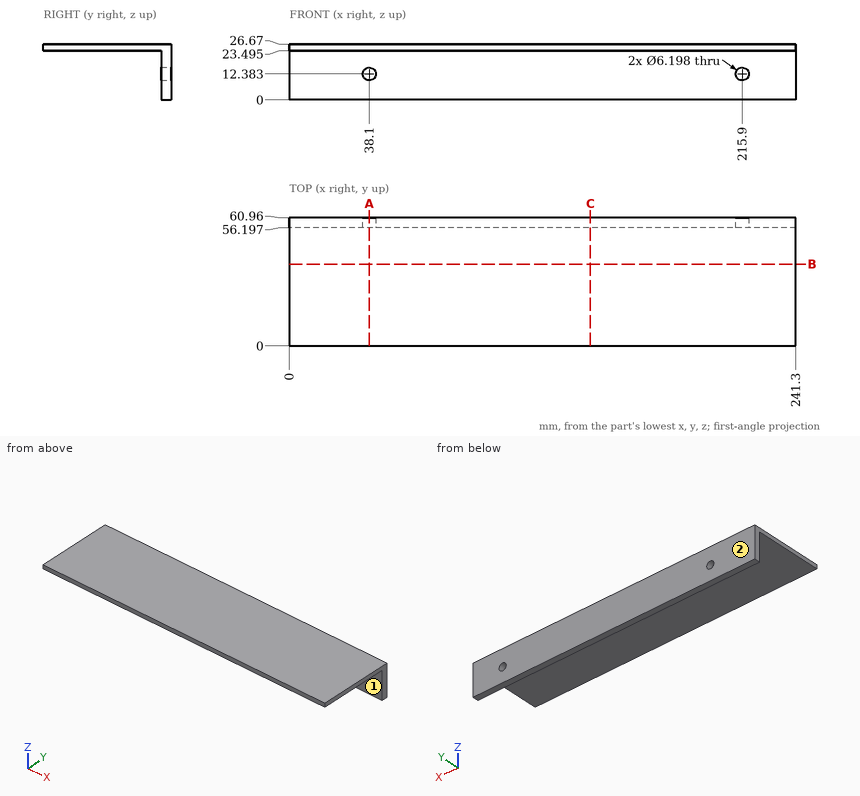
Verification items for this drawing (mm, ordinates from the low corner). A direction names the side the tool comes from. Give positions to 0.01 mm unless a question says otherwise; leave off trailing zeros. Loops run counter-clockwise (first coordinate to the right, second up) from the corner with the lowest first, then second, coordinate; pieces in that order, holes last. Notation, with made-up numbers: (66, 72.5) - (122, 72.5) arc R29 cw to (122, 99.5) - close; hole circle Ø8 at (76, 74.25). An arc over 180 degrees is marked (long way). Write item = value, one per line. Start each with the question number.
Q1. Tool access check on the marked faces 1 and 2. Record the directions out of +Z, -Z, +X, -X, +Y, -Y that give a thin tool (end or side, any length) a straight path to the whole face; none if there is none.
Q2. Thickness scan on line 1 (Z direction, x = 215.9, y = 58.9); line 2 (Y direction, x = 120, z = 3.25); line 3 (Z direction, x = 59, y = 31.5) (1 decimal). Record the ranges inside material, lowest first.
Q3. Cross-section at C-C, the plane x = 143.5. Enter the section's corners in (y, z) (1 decimal).
Q4. Depth check by flat-ended pin: P1, Ø12, axis at x = 144.5, y = 21, coming from the -Z side (1 decimal); P2, Ø12, axis at y = 54.5, z = 11, coming from the +X side; P3, Ø8, axis at x = 215.9, z = 12.38, coming from the -Y side. Enter the tip coordinate at first touch or a pass-through.
Q5. Cross-section at A-A, the plane x = 38.1. Enter the section's corners in (y, z) (1 decimal).
Q6. Cross-section at B-B, the plane y = 39. Enter the section's corners in (x, z) (1 decimal).
Answer key:
q1.face_1 = -Z, +X, -X, -Y
q1.face_2 = +Z, -Z, +X, -X, +Y
q2.line_1 = 0 to 9.28, 15.48 to 26.67
q2.line_2 = 56.2 to 60.96
q2.line_3 = 23.5 to 26.7
q3.outline = (0, 23.5) - (56.2, 23.5) - (56.2, 0) - (61, 0) - (61, 26.7) - (0, 26.7) - close
q4.P1 = 23.5
q4.P2 = 241.3
q4.P3 = 56.2
q5.outline = (0, 23.5) - (56.2, 23.5) - (56.2, 15.5) - (61, 15.5) - (61, 26.7) - (0, 26.7) - close; (56.2, 0) - (61, 0) - (61, 9.3) - (56.2, 9.3) - close
q6.outline = (0, 23.5) - (241.3, 23.5) - (241.3, 26.7) - (0, 26.7) - close
